Source: CAD feature listing. Evaluate the final solid. Frame: model axes, mm. A direction names the side the tool comes from. Round coordinates to 2 decimals unless told otherwise and drop trailing zeros. Write each loop counter-clockwise with the first axis right and the second up, starting at its lowest first coordinate (ties: lowest second). Pieces come first, ordered by that corner, then holes.
Autodesk Inventor part; units mm, degrees
ref_plane "GRIFF_XY" through (0, 0, 0) normal (1, 0, 0) x (0, 0, -1)
ref_plane "GRIFF_YZ" through (0, 0, 0) normal (0, 0, -1) x (0, 1, 0)
ref_plane "GRIFF_ZX" through (0, 0, 0) normal (0, 1, 0) x (1, 0, 0)
sketch "Sketch_1" plane through (0, 0, 0) normal (1, 0, 0) x (0, 1, 0)
  arc A0 (10.1247, 7.5) -> (12.3488, -2.5033) centre (0, 0) ccw
  arc A1 (14.799, -0.5) -> (12.3488, -2.5033) centre (14.799, -3) ccw
  line L0 (14.799, -0.5) -> (46, -0.5)
  line L1 (46, -0.5) -> (46, 7.5)
  line L2 (46, 7.5) -> (10.1247, 7.5)
extrude "Extrusion1" add sketch "Sketch_1" along normal mid plane 14
sketch "Sketch_2" plane through (0, 0, 0) normal (0, 0, 1) x (1, 0, 0)
  line L0 (-7, -24.7) -> (7, -24.7)
  line L1 (7, -24.7) -> (7, 16.5)
  line L2 (7, 16.5) -> (6.5, 16.5)
  arc A0 (6.5, 16.5) -> (3, 13) centre (6.5, 13) ccw
  line L3 (3, 13) -> (3, -21.7)
  line L4 (3, -21.7) -> (-3, -21.7)
  line L5 (-3, -21.7) -> (-3, 13)
  arc A1 (-3, 13) -> (-6.5, 16.5) centre (-6.5, 13) ccw
  line L6 (-6.5, 16.5) -> (-7, 16.5)
  line L7 (-7, 16.5) -> (-7, -24.7)
extrude "Extrusion2" cut sketch "Sketch_2" along normal mid plane 30
sketch "Sketch_3" plane through (0, 0, 8.5) normal (0, 0, 1) x (1, 0, 0)
  line L0 (7, 16.5) -> (7.5, 16.5)
  line L1 (7.5, 16.5) -> (8, 17)
  line L2 (8, 17) -> (8, 45.5)
  line L3 (8, 45.5) -> (7.5, 46)
  line L4 (7.5, 46) -> (7, 46)
  line L5 (7, 46) -> (7, 16.5)
extrude "Extrusion3" add sketch "Sketch_3" against normal blind 10
sketch "Sketch_4" plane through (0, 0, 8.5) normal (0, 0, 1) x (1, 0, 0)
  line L0 (-8, 17) -> (-7.5, 16.5)
  line L1 (-7.5, 16.5) -> (-7, 16.5)
  line L2 (-7, 16.5) -> (-7, 46)
  line L3 (-7, 46) -> (-7.5, 46)
  line L4 (-7.5, 46) -> (-8, 45.5)
  line L5 (-8, 45.5) -> (-8, 17)
extrude "Extrusion4" add sketch "Sketch_4" against normal blind 10
sketch "Sketch_5" plane through (0, 0, 0) normal (1, 0, 0) x (0, 1, 0)
  line L0 (32, -0.5) -> (32, 7.5)
  line L1 (32, 7.5) -> (34.5, 7.5)
  line L2 (34.5, 7.5) -> (34, 7)
  line L3 (34, 7) -> (34, 0)
  line L4 (34, 0) -> (34.5, -0.5)
  line L5 (34.5, -0.5) -> (32, -0.5)
  line L6 (32, -0.5) -> (32, 7.5)
revolve "Revolution1" cut sketch "Sketch_5" angle 360 about axis through (0, 32, -0.5) along (0, 0, -1)
sketch "Sketch6" plane through (-3, 10.1247, 7.5) normal (0, 0, 1) x (1, 0, 0)
  point P0 (3, 14.8753)
hole "Hole1" at (0, 25, 7.5) direction (0, 0, -1) diameter 4.134 depth 8
sketch "Sketch7" plane through (-3, 10.1247, 7.5) normal (0, 0, 1) x (1, 0, 0)
  point P0 (3, 28.8753)
hole "Hole2" at (0, 39, 7.5) direction (0, 0, -1) diameter 4.134 depth 8
sketch "Sketch_9" plane through (0, 0, 0) normal (1, 0, 0) x (0, 1, 0)
  arc A0 (-11.5335, 7.2069) -> (-12.1177, 6.1743) centre (0, 0) ccw
  line L0 (-12.1177, 6.1743) -> (0, 0)
  line L1 (0, 0) -> (-11.5335, 7.2069)
extrude "Extrusion5" add sketch "Sketch_9" along normal mid plane 2
ref_plane "GRIFF_XY" through (0, 0, 0) normal (1, 0, 0) x (0, 0, -1)
ref_plane "GRIFF_YZ" through (0, 0, 0) normal (0, 0, -1) x (0, 1, 0)
ref_plane "GRIFF_ZX" through (0, 0, 0) normal (0, 1, 0) x (1, 0, 0)
properties part number "1310164 DHRS-32-A---(Griff)"
Q1. Section query C-C, the plane y = 32. Output: boundary loops of the cut face in (x, z), and give its area (3 significant figures).
Q2. Line query: line 1 (X direction, y = 25, z = 1.25); line 2 (Y direction, x = -1.25, z = 0.5); line 3 (X direction, y = 32, z = 5.75). Output: solid intervals per line, ascending.
Q3. Pin query (flat end, axial travel): P1, Ø1.1, axis at x = 7.5, y = 28, coming from the -Z side; P2, Ø2, axis at y = 12, z = -4, coming from the -X side; P3, Ø5.5, axis at x = 0, y = 25, coming from the -Z side; P4, Ø1.5, axis at x = 4, y = 0.5, coming from the -Z side. Return the tip coordinate at first contact, or that it passes through.
Q4. Section query A-A, the plane y = 25. Output: boundary loops of the cut face in (x, z), and give its area (3 significant figures).
Q5. Section query D-D, the plane z = -8.25. Output: boundary loops of the cut face in (x, y).
Q6. Set-up query: faces 1 (the face through (-1, -11.4, 6.5)), 2 (the face through (-7, 31, -1)), 3 (the face through (-3, 0, 0)). Return all of +Z, -Z, +X, -X, +Y, -Y with unobstructed straight access to the full face (end or side cutting, diameter ignored); none if empty.
Q7. Section query B-B, the plane z = 2.5. Output: boundary loops of the cut face in (x, y).
Filled in:
1. outline: (-8, -1.5) - (-7, -1.5) - (-7, -0.5) - (-2.5, -0.5) - (-2, 0) - (-2, 7) - (-2.5, 7.5) - (-7, 7.5) - (-7, 8.5) - (-8, 8.5) - close; (2, 0) - (2.5, -0.5) - (7, -0.5) - (7, -1.5) - (8, -1.5) - (8, 8.5) - (7, 8.5) - (7, 7.5) - (2.5, 7.5) - (2, 7) - close
1. area: 99.5 mm2
2. line 1: x = -8 to -2.07, 2.07 to 8
2. line 2: y = -12.59 to 23.35, 26.65 to 30.44, 33.56 to 37.35, 40.65 to 46
2. line 3: x = -8 to -2, 2 to 8
3. P1: stops at z = -1.5
3. P2: stops at x = -3
3. P3: stops at z = -0.5
3. P4: passes through
4. outline: (-8, -1.5) - (-7, -1.5) - (-7, -0.5) - (-2.07, -0.5) - (-2.07, 7.5) - (-7, 7.5) - (-7, 8.5) - (-8, 8.5) - close; (2.07, -0.5) - (7, -0.5) - (7, -1.5) - (8, -1.5) - (8, 8.5) - (7, 8.5) - (7, 7.5) - (2.07, 7.5) - close
4. area: 98.9 mm2
5. outline: (-3, -9.52) - (3, -9.52) - (3, 9.52) - (-3, 9.52) - close
6. face 1: +Z, -X, -Y
6. face 2: -Z, +Y, -Y
6. face 3: +Z, -Z, -X, -Y
7. outline: (-8, 17) - (-7.5, 16.5) - (-6.5, 16.5) arc R3.5 cw to (-3, 13) - (-3, -12.35) - (3, -12.35) - (3, 13) arc R3.5 cw to (6.5, 16.5) - (7.5, 16.5) - (8, 17) - (8, 45.5) - (7.5, 46) - (-7.5, 46) - (-8, 45.5) - close; hole circle Ø4.13 at (0, 25); hole circle Ø4.13 at (0, 39); hole circle Ø4 at (0, 32)
